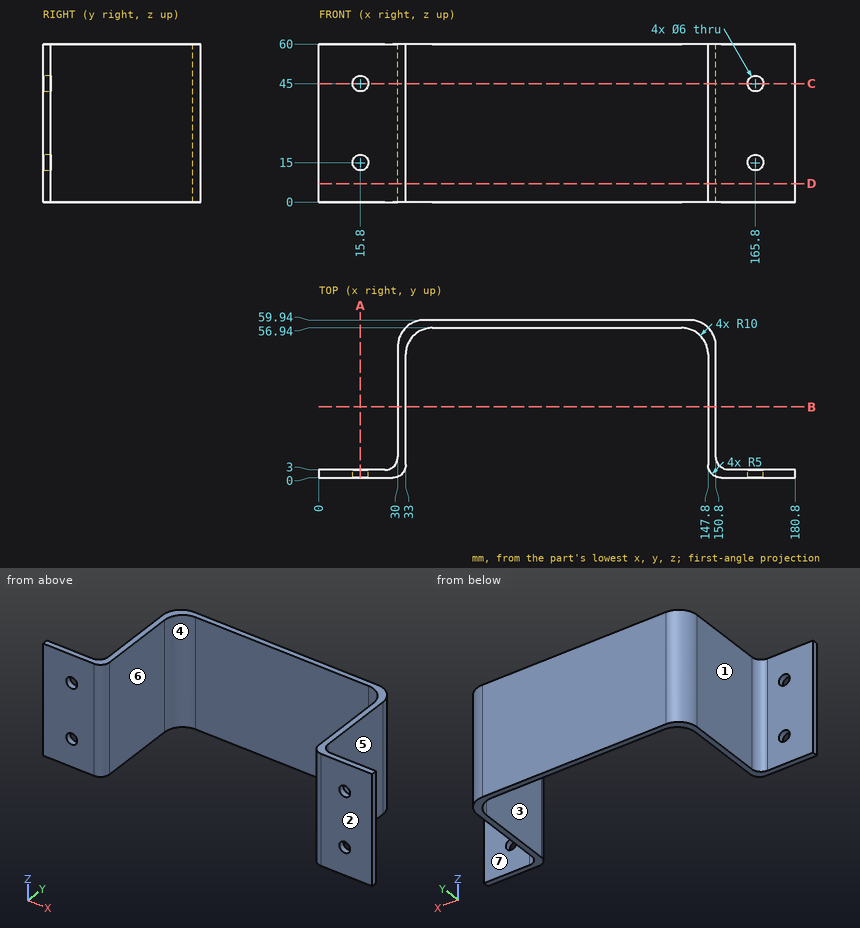
Check sheet for the drawn part. Datum: minimum x, y, z corner. Units: mm. A direction names the side the tool comes from. Round coordinates to 2 decimals unless told otherwise and drop trailing zeros. Loops run counter-clockwise (first coordinate to the right, second up) from the corner with the lowest first, then second, coordinate; pieces in that order, holes last.
Item 1: Thickness scan on line 1 (Z direction, x = 165.8, y = 1.5); line 2 (X direction, y = 38.5, z = 50.5); line 3 (X direction, y = 1.6, z = 45). Record the ranges inside material, lowest first.
Item 2: Cross-section at C-C on z = 45. Record the boundary of the cut face in (x, y), then the cut area to 3 significant figures.
Item 3: Gauge pin test, flat ends, axial feed: pin 1 (10 mm diameter, centred on x = 52, z = 47.5, fed in from -Y); pin 2 (12.5 mm diameter, centred on y = 37, z = 16, fed in from +X); pin 3 (7.5 mm diameter, centred on x = 12.5, z = 15.5, fed in from +Y). Record the tip position at first contact, or that the pin passes through.
Item 4: Mould release check, pull along X, two halves, no side actions. Record for the marked faces 4, 5, 6 and 7: pulls with the +X half, pulls with the -X half, needs draft (parallel to the pull), parting line crosses it, or undercut.
Item 5: Cross-section at A-A on x = 15.8. Record the boundary of the cut face in (y, z), then the cut area to 3 significant figures.
Item 6: Cross-section at B-B on y = 27. Record the boundary of the cut face in (x, z).
Item 7: Cross-section at D-D on z = 7. Record the boundary of the cut face in (x, y), then the cut area to 3 significant figures.
Item 8: Access from +Z, -Z, +X, -X, +Y, -Y to the whole of each face (thin tool, end or side, straight path). Record for the marked faces 1, 2 and 3.
Answer sheet:
1. line 1: z = 0 to 12, 18 to 42, 48 to 60
1. line 2: x = 30 to 33, 147.8 to 150.8
1. line 3: x = 0 to 12.8, 18.8 to 31.67, 149.13 to 162.8, 168.8 to 180.8
2. outline: (0, 0) - (12.8, 0) - (12.8, 3) - (0, 3) - close; (18.8, 0) - (28, 0) arc R5 ccw to (33, 5) - (33, 46.94) arc R10 cw to (43, 56.94) - (137.8, 56.94) arc R10 cw to (147.8, 46.94) - (147.8, 5) arc R5 ccw to (152.8, 0) - (162.8, 0) - (162.8, 3) - (155.8, 3) arc R5 cw to (150.8, 8) - (150.8, 49.94) arc R10 ccw to (140.8, 59.94) - (40, 59.94) arc R10 ccw to (30, 49.94) - (30, 8) arc R5 cw to (25, 3) - (18.8, 3) - close; (168.8, 0) - (180.8, 0) - (180.8, 3) - (168.8, 3) - close
2. area: 848 mm2
3. pin 1: stops at y = 56.94
3. pin 2: stops at x = 150.8
3. pin 3: stops at y = 3
4. face 4: undercut
4. face 5: pulls with the +X half
4. face 6: undercut
4. face 7: needs draft
5. outline: (0, 0) - (3, 0) - (3, 12) - (0, 12) - close; (0, 18) - (3, 18) - (3, 42) - (0, 42) - close; (0, 48) - (3, 48) - (3, 60) - (0, 60) - close
5. area: 144 mm2
6. outline: (30, 0) - (33, 0) - (33, 60) - (30, 60) - close; (147.8, 0) - (150.8, 0) - (150.8, 60) - (147.8, 60) - close
7. outline: (0, 0) - (28, 0) arc R5 ccw to (33, 5) - (33, 46.94) arc R10 cw to (43, 56.94) - (137.8, 56.94) arc R10 cw to (147.8, 46.94) - (147.8, 5) arc R5 ccw to (152.8, 0) - (180.8, 0) - (180.8, 3) - (155.8, 3) arc R5 cw to (150.8, 8) - (150.8, 49.94) arc R10 ccw to (140.8, 59.94) - (40, 59.94) arc R10 ccw to (30, 49.94) - (30, 8) arc R5 cw to (25, 3) - (0, 3) - close
7. area: 884 mm2
8. face 1: +Z, -Z, -X, +Y
8. face 2: +Z, -Z, +X, -X, -Y
8. face 3: +Z, -Z, -Y
